Verification items for the finished model (mm, model axes). A direction names the side the tool comes from. Round coordinates to 2 decimals unless told otherwise and drop trailing zeros. Order: outer loops, then holes, each group sorted by start corner. A loop starts at its lowest first (then second) coordinate and runs counter-clockwise, first axis right, second up. Notation, with made-up numbers: M 27.5,51 L 72.5,51 A16 cw 72.5,57 Z; hole C 76.5,26.25 d9. An arc over 180 degrees is marked long. Use one line per item in the form item = value. Start each with the question number.
Item 1: Cross-section at A-A on z = 751. Enter the section's corners in (x, y).
Item 2: Cross-section at B-B on x = 12.75. Enter the section's corners in (y, z), then the cut area to 3 significant figures.
Item 3: Go/stop test with flat-tipped pins: pin 1 Ø12 at (x, y) = (1.5, 19) entering from +Z; pin 2 Ø5 at (y, z) = (-5.5, 319) entering from +X; pin 3 Ø3 at (x, z) = (8, 1048.5) entering from +Y. Record where each tip stops, or that it passes through.
Item 4: Cross-section at C-C on y = 12. Enter the section's corners in (x, z), then the cut area to 3 significant figures.
Item 5: Tool access check on faces 1 (the flat face through (-2.41, 11, 690)), 2 (the flat face through (-3.59, 0.41, -6.58)). Record the directions out of +Z, -Z, +X, -X, +Y, -Y that give a thin tool (end or side, any length) a straight path to the whole face; none if there is none.
Item 6: Thickness scan on probe 1 along X at (y, z) = (26, 892.5); probe 2 along Y at (x, z) = (-5.5, 103.5); probe 3 along Y at (x, z) = (11.5, 393). Record the ranges inside material, lowest first. Write a range as [from, to].
Autodesk Inventor part; units mm, degrees
ref_plane "Start Plane" through (0, 0, -24.2929) normal (0, 0, 1) x (1, 0, 0)
ref_plane "End Plane" through (0, 0, 1424.2929) normal (0, 0, 1) x (1, 0, 0)
ref_plane "Work Plane11" through (7.59, -17.6536, 1424.6464) normal (0, 0.7071, 0.7071) x (1, 0, 0)
ref_plane "Start Plane" through (0, 0, -24.2929) normal (0, 0, 1) x (1, 0, 0)
ref_plane "End Plane" through (0, 0, 1424.2929) normal (0, 0, 1) x (1, 0, 0)
sketch "Sketch" plane through (0, 0, 0) normal (0, 0, 1) x (1, 0, 0)
  line L0 (-2.41, 28.7) -> (-2.41, -7.3)
  line L1 (-7.41, 32.7) -> (-6.41, 32.7)
  line L2 (-7.41, -17.3) -> (-7.41, 32.7)
  line L3 (22.59, -17.3) -> (-7.41, -17.3)
  line L4 (22.59, -16.3) -> (22.59, -17.3)
  line L5 (2.59, -12.3) -> (18.59, -12.3)
  arc A0 (-2.41, -7.3) -> (2.59, -12.3) centre (2.59, -7.3) ccw
  arc A1 (-2.41, 28.7) -> (-6.41, 32.7) centre (-6.41, 28.7) ccw
  arc A2 (22.59, -16.3) -> (18.59, -12.3) centre (18.59, -16.3) ccw
  line L6 (0, 43.6941) -> (0, -27.4657) construction
  line L7 (-13.5757, 0) -> (29.5841, 0) construction
  point P0 (-2.41, 32.7)
  point P1 (-2.41, -12.3)
  point P2 (22.59, -12.3)
  dimension "d4" = 30
  dimension "d6" = 50
  dimension "d8" = 5
  dimension "d10" = 5
  dimension "d17" = 5
  dimension "d18" = 4
  dimension "d19" = 17.3
  dimension "d20" = 7.41
extrude "Body" add sketch "Sketch" along normal up to surface (1448.5858 mm away) from surface at -24.2929
sketch "Sketch3" plane through (0, 0, 0) normal (0, 0, 1) x (1, 0, 0)
  line L0 (0, 0) -> (10, 0)
ref_plane "Work Plane10" through (0, 0, 0) normal (0, -1, 0) x (1, 0, 0)
sketch "Sketch4" plane through (0, 0, 0) normal (0, -1, 0) x (1, 0, 0)
  line L0 (-2, -24.2929) -> (12, -24.2929)
  line L1 (-2, 1424.2929) -> (12, 1424.2929)
  dimension "d24" = 1448.5858
ref_plane "Work Plane11" through (7.59, -17.6536, 1424.6464) normal (0, 0.7071, 0.7071) x (1, 0, 0)
split "Split1" plane through (7.59, -17.6536, 1424.6464) removes the side toward (0, 0.7071, 0.7071)
ref_plane "Work Plane12" through (7.59, -17.6536, -24.6464) normal (0, 0.7071, -0.7071) x (1, 0, 0)
split "Split2" plane through (7.59, -17.6536, -24.6464) removes the side toward (0, 0.7071, -0.7071)
equation "\"d4\" = b"
equation "\"d6\" = ParH"
equation "\"d17\" = R"
equation "\"d18\" = R1"
equation "\"d19\" = ex"
equation "\"d20\" = ey"
equation "\"d11\" = G_L"
equation "\"b\" = 30"
equation "\"ParT\" = 5"
equation "\"R1\" = 4"
equation "\"G_L\" = d24"
equation "\"ParH\" = 50"
equation "\"R\" = 5"
equation "\"ey\" = 7.41"
equation "\"ex\" = 17.3"
equation "\"G_OFFSET_START\" = 24.29289"
equation "\"G_OFFSET_END\" = 24.29289"
equation "\"d21\" = -G_OFFSET_START"
equation "\"d22\" = G_OFFSET_END + B_L"
properties part number "ISO 657-2 - 50x 30x 5-1448.59" material "Steel, Mild"
Output values:
q1.outline = M -7.41,-17.3 L 22.59,-17.3 L 22.59,-16.3 A4 ccw 18.59,-12.3 L 2.59,-12.3 A5 cw -2.41,-7.3 L -2.41,28.7 A4 ccw -6.41,32.7 L -7.41,32.7 Z
q2.outline = M -17.3,-24.29 L -12.3,-19.29 L -12.3,1419.29 L -17.3,1424.29 Z
q2.area = 7,220 mm2
q3.pin_1 = 1392.54
q3.pin_2 = -2.36
q3.pin_3 = -12.3
q4.outline = M -7.41,5.01 L -2.41,5.01 L -2.41,1394.99 L -7.41,1394.99 Z
q4.area = 6,950 mm2
q5.face_1 = +Z, -Z, +X, +Y
q5.face_2 = -Z, +X, -X, +Y
q6.probe_1 = [-7.41, -2.41]
q6.probe_2 = [-17.3, 32.6]
q6.probe_3 = [-17.3, -12.3]
